Here's the drawing with two shaded views (mm, measured from the low corner). I have some questions. A direction names the side the tool comes from. Coordinates: 2 decimals unless noted, no trailing zeros. Loops run counter-clockwise (first coordinate to the right, second up) from the corner with the lowest first, then second, coordinate; pieces in that order, holes last. Notation, with made-up numbers: (55, 19.25) -> (88, 19.25) arc R12 cw to (88, 42.25) -> close; hole circle Ø8 at (-37.75, -8). An arc over 180 degrees is marked (long way). Answer as a JSON object with one key per item and string values. Group by question number.
1) I want a section at C-C (x = 35.5). Write out the boundary of the cut face in (y, z).
2) I want a section at B-B (y = 55). Write out the boundary of the cut face in (x, z).
3) Which directions (+Z, -Z, +X, -X, +Y, -Y) give clear straight access to the entire face, cutting with the end or side of a thin tool? Please do the marked faces 1 and 2.
4) I'm going to push flat-ended pins straight in: pin 1 (15.5 mm diameter, centred on y = 42, z = 33, fed in from -X); pin 2 (4 mm diameter, centred on y = 42, z = 9.5, fed in from -X); pin 3 (6 mm diameter, centred on y = 46.5, z = 50, fed in from -X). Where does each tip first touch, or does it pass through?
5) I need wall thicknesses on probe 1 along X at (y, z) = (42, 32); probe 2 along Z at (x, y) = (44.5, 61); probe 3 along X at (y, z) = (53, 18). Which ranges of each line are inside material? Lowest first, please. Write a range as [from, to].
6) I want a section at A-A (z = 32.5). Write out the boundary of the cut face in (x, y), then the cut area to 3 significant figures.
7) If we mould it in two halves opening along Z, with no side actions, what happens to the marked faces 3, 4, 5 and 6? For each: +Z half, -Z half, draft (parallel to the pull), parting line (faces both ways), or undercut.
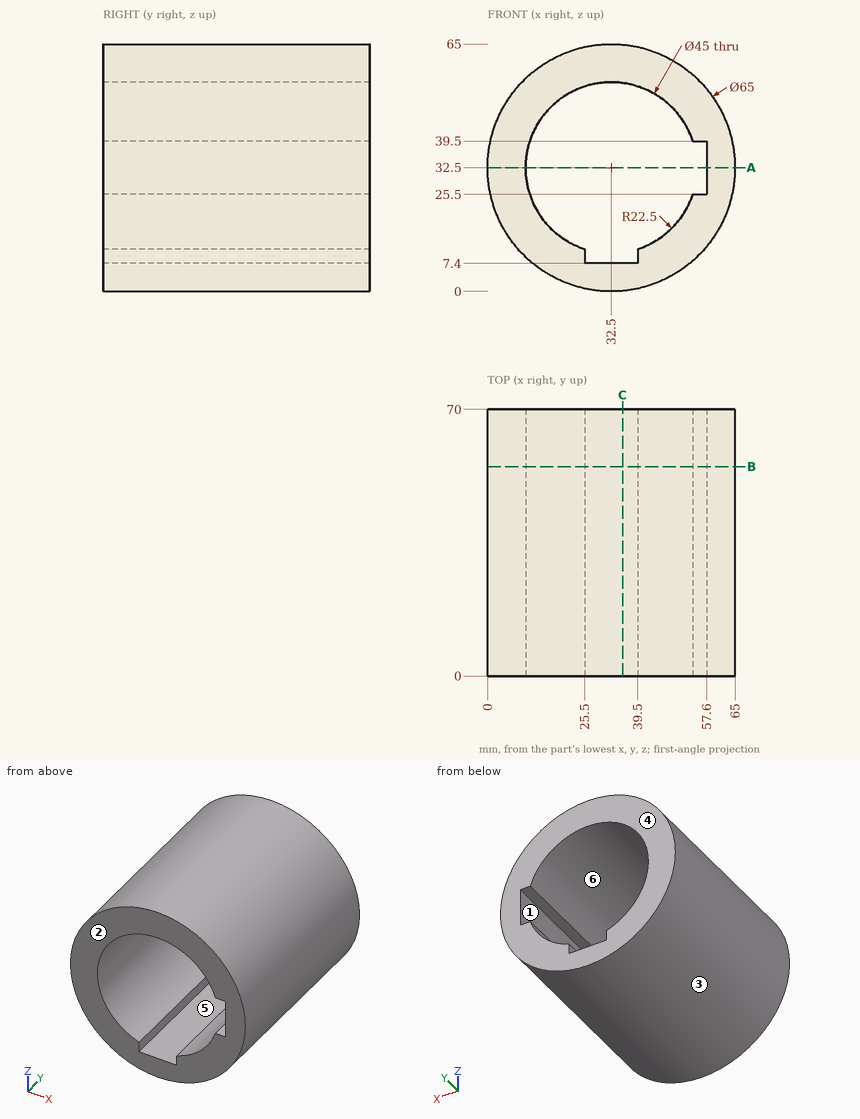
Determined:
{
 "1": {"outline": "(0, 0.14) -> (70, 0.14) -> (70, 7.4) -> (0, 7.4) -> close; (0, 54.8) -> (70, 54.8) -> (70, 64.86) -> (0, 64.86) -> close"},
 "2": {"outline": "circle Ø65 at (32.5, 32.5); hole (25.5, 7.4) -> (39.5, 7.4) -> (39.5, 11.12) arc R22.5 ccw to (53.88, 25.5) -> (57.6, 25.5) -> (57.6, 39.5) -> (53.88, 39.5) arc R22.5 ccw (long way) to (25.5, 11.12) -> close"},
 "3": {"face 1": "+Y, -Y", "face 2": "+Z, -Z, +X, -X, -Y"},
 "4": {"pin 1": "x = 0", "pin 2": "x = 7.7", "pin 3": "x = 3.41"},
 "5": {"probe 1": "[0, 10.01], [57.6, 65]", "probe 2": "[2.3, 13.47], [51.53, 62.7]", "probe 3": "[3.41, 15.3], [49.7, 61.59]"},
 "6": {"outline": "(0, 0) -> (10, 0) -> (10, 70) -> (0, 70) -> close; (57.6, 0) -> (65, 0) -> (65, 70) -> (57.6, 70) -> close", "area": "1,220 mm^2"},
 "7": {"face 3": "parting line", "face 4": "draft", "face 5": "undercut", "face 6": "undercut"}
}
